Can you work these out from the model? Positions are in its coordinate system, mm. A direction names the side the tool comes from. Give positions to 0.01 mm unless a question says otherwise; leave off trailing zeros. Write each loop counter-clockwise with the first axis right and the second up, starting at its lowest first coordinate (ties: lowest second). Pieces come first, ordered by that corner, then holes. Notation, with made-up numbers: M 30.5,71.25 L 62.5,71.25 A17 ccw 62.5,100.25 Z; hole C 62.5,14.25 d7. An arc over 180 degrees is marked long. Write each question's results on one line, items separated by ' | '.
from build123d import *

# Parameters (mm, degrees)
SKETCH1_W           = 130
SKETCH1_H           = 130
BOSS_EXTRUDE1_DEPTH = 4
CUT_EXTRUDE1_DEPTH  = 4
SKETCH6_W           = 60.337998114
SKETCH6_H           = 11.352835906
BOSS_EXTRUDE2_DEPTH = 2
CIRPATTERN1_COUNT   = 4
BOSS_EXTRUDE3_START = -2
BOSS_EXTRUDE3_DEPTH = 2
CIRPATTERN2_COUNT   = 4
SKETCH10_R          = 1.5
CUT_EXTRUDE2_DEPTH  = 93.010868923
CIRPATTERN3_COUNT   = 4


with BuildPart() as part:
    # Sketch1 → Boss-Extrude1 (new body)
    with BuildSketch(Plane(origin=(0, 0, 0), x_dir=(1, 0, 0), z_dir=(0, 1, 0))):
        Rectangle(SKETCH1_W, SKETCH1_H)
    extrude(amount=BOSS_EXTRUDE1_DEPTH)

    # Sketch5 → Cut-Extrude1 (cut)
    with BuildSketch(Plane(origin=(0, 4, 0), x_dir=(1, 0, 0), z_dir=(0, 1, 0))):
        with BuildLine():
            ThreePointArc((29.836037364, 44.227066084), (0, 53.35), (-29.836037364, 44.227066084))
            ThreePointArc((-29.836037364, 44.227066084), (-39.783378413, 39.783378413), (-44.227066084, 29.836037364))
            ThreePointArc((-44.227066084, 29.836037364), (-53.35, 0), (-44.227066084, -29.836037364))
            ThreePointArc((-44.227066084, -29.836037364), (-39.783378413, -39.783378413), (-29.836037364, -44.227066084))
            ThreePointArc((-29.836037364, -44.227066084), (0, -53.35), (29.836037364, -44.227066084))
            ThreePointArc((29.836037364, -44.227066084), (39.783378413, -39.783378413), (44.227066084, -29.836037364))
            ThreePointArc((44.227066084, -29.836037364), (53.35, 0), (44.227066084, 29.836037364))
            ThreePointArc((44.227066084, 29.836037364), (39.783378413, 39.783378413), (29.836037364, 44.227066084))
        make_face()
    extrude(amount=-CUT_EXTRUDE1_DEPTH, mode=Mode.SUBTRACT)

    # Sketch6 → Boss-Extrude2 (add)
    with BuildSketch(Plane.XZ):
        with Locations((0, 48.86626436)):
            Rectangle(SKETCH6_W, SKETCH6_H)
    boss_extrude2 = extrude(amount=-BOSS_EXTRUDE2_DEPTH)

    # CirPattern1: Boss-Extrude2 ×4 about axis
    cirpattern1_axis = Axis((0, 0, 0), (0, 1, 0))
    for i in range(1, CIRPATTERN1_COUNT):
        add(boss_extrude2.rotate(cirpattern1_axis, i * 360 / CIRPATTERN1_COUNT))

    # Sketch9 → Boss-Extrude3 (add)
    with BuildSketch(Plane.XZ.offset(BOSS_EXTRUDE3_START)):
        with BuildLine():
            Line((-30.168999057, 44.20512878), (-30.168999057, 43.189846407))
            ThreePointArc((-30.168999057, 43.189846407), (-39.067728141, 39.067728141), (-43.189846407, 30.168999057))
            Line((-43.189846407, 30.168999057), (-44.20512878, 30.168999057))
            ThreePointArc((-44.20512878, 30.168999057), (-39.783378413, 39.783378413), (-30.168999057, 44.20512878))
        make_face()
    boss_extrude3 = extrude(amount=BOSS_EXTRUDE3_DEPTH)

    # CirPattern2: Boss-Extrude3 ×4 about axis
    cirpattern2_axis = Axis((0, 0, 0), (0, 1, 0))
    for i in range(1, CIRPATTERN2_COUNT):
        add(boss_extrude3.rotate(cirpattern2_axis, i * 360 / CIRPATTERN2_COUNT))

    # Sketch10 → Cut-Extrude2 (cut, through all)
    with BuildSketch(Plane(origin=(0, 4, 0), x_dir=(1, 0, 0), z_dir=(0, 1, 0))):
        with Locations(Location((-63, 63, 0), (0, 0, 270))):
            Circle(SKETCH10_R)
        with Locations(Location((-57, 63, 0), (0, 0, 270))):
            Circle(SKETCH10_R)
        with Locations(Location((-63, 57, 0), (0, 0, 270))):
            Circle(SKETCH10_R)
    cut_extrude2 = extrude(amount=-CUT_EXTRUDE2_DEPTH, mode=Mode.SUBTRACT)

    # CirPattern3: Cut-Extrude2 ×4 about axis
    cirpattern3_axis = Axis((0, 0, 0), (0, 1, 0))
    for i in range(1, CIRPATTERN3_COUNT):
        add(cut_extrude2.rotate(cirpattern3_axis, i * 360 / CIRPATTERN3_COUNT), mode=Mode.SUBTRACT)


solid = part.part
Item 1: I want a section at C-C, the plane x = 63. Please give me the cut outline in (y, z).
Geometry says:
outline: M 0,-65 L 4,-65 L 4,-64.5 L 0,-64.5 Z; M 0,-61.5 L 4,-61.5 L 4,-58.5 L 0,-58.5 Z; M 0,-55.5 L 4,-55.5 L 4,55.5 L 0,55.5 Z; M 0,58.5 L 4,58.5 L 4,61.5 L 0,61.5 Z; M 0,64.5 L 4,64.5 L 4,65 L 0,65 Z
Item 2: Thinking about a two-plate mould opening in Z: for faces 1 (the face through (65, 2, 1)), 2 (the face through (-62.55, 2.03, -61.57)), 3 (the face through (-1, 2, 65)), which applies, +Z half, -Z half, draft (parallel to the pull), parting line (faces both ways), or undercut?
Geometry says:
face 1: draft | face 2: undercut | face 3: +Z half
Item 3: I want a section at A-A, the plane z = 57. Please give me the cut outline in (x, y), and give its area (3 significant figures).
Geometry says:
outline: M -65,0 L -64.5,0 L -64.5,4 L -65,4 Z; M -61.5,0 L 61.5,0 L 61.5,4 L -61.5,4 Z; M 64.5,0 L 65,0 L 65,4 L 64.5,4 Z | area: 496 mm2
Item 4: If I drill on line 1 (Z direction, x = 63, y = 2.9); line 2 (X direction, y = 3.05, z = 57), over which ranges is the centre line in solid material (lowest first)? Write a range as from..to.
Geometry says:
line 1: z = -65..-64.5, -61.5..-58.5, -55.5..55.5, 58.5..61.5, 64.5..65 | line 2: x = -65..-64.5, -61.5..61.5, 64.5..65
Item 5: I want a section at D-D, the plane x = 26.5. Please give me the cut outline in (y, z).
Geometry says:
outline: M 0,-65 L 4,-65 L 4,-46.3 L 2,-46.3 L 2,-43.19 L 0,-43.19 Z; M 0,43.19 L 2,43.19 L 2,46.3 L 4,46.3 L 4,65 L 0,65 Z
Item 6: I'm going to push flat-ended pins straight in: pin 1 (5 mm diameter, centred on x = -57, z = -63, fed in from -Y); pin 2 (1.8 mm diameter, centred on x = 57, z = -63, fed in from +Y); pin 3 (8 mm diameter, centred on x = -41, z = -9.5, fed in from +Y). Where does each tip first touch, or does it pass through?
Geometry says:
pin 1: stops at y = 0 | pin 2: passes through | pin 3: stops at y = 2
Item 7: For faces 4 (the face through (0.44, 3.01, -53.35)), 5 (the face through (-38.968, 1.014, 39.166)), 6 (the face through (-59, 4, -1)), which set-ups out of +Z, -Z, +X, -X, +Y, -Y let a thin tool reach every point of the face, with its end or its side?
Geometry says:
face 4: +Y | face 5: +Y, -Y | face 6: +Z, -Z, +X, -X, +Y
Item 8: I want a section at B-B, the plane y = 1.4. Give the number of separate pieces and of enclosed holes in the cut face, and give its area (3 significant figures).
Geometry says:
separate pieces: 1 | enclosed holes: 13 | area: 9,520 mm2
